from build123d import *

# Parameters (mm, degrees)
EXTRUDE_1_DEPTH           = 70
SKETCH_4_R                = 2.5
EXTRUDE_2_DEPTH           = 10
M5X0_8_TAPPED_HOLE1_D     = 4.2
M5X0_8_TAPPED_HOLE1_DEPTH = 12.4
M5X0_8_TAPPED_HOLE1_TIP   = 1.2618073


with BuildPart() as part:
    # 草圖1 → 填料-伸長1 (new body)
    with BuildSketch(Plane.XY):
        Polygon((-2.020725942, 3.5), (-4.041451884, 0), (-2.020725942, -3.5), (2.020725942, -3.5), (4.041451884, 0), (2.020725942, 3.5), align=None)
    extrude(amount=EXTRUDE_1_DEPTH)

    # 草圖4 → 填料-伸長2 (add)
    with BuildSketch(Plane(origin=(0, 0, 0), x_dir=(-1, 0, 0), z_dir=(0, 0, -1))):
        Circle(SKETCH_4_R)
    extrude(amount=EXTRUDE_2_DEPTH)

    # M5x0.8 Tapped Hole1
    with Locations(Plane.XY.offset(70)):
        with Locations((0, 0)):
            Hole(M5X0_8_TAPPED_HOLE1_D / 2, depth=M5X0_8_TAPPED_HOLE1_DEPTH)
            with Locations((0, 0, -(M5X0_8_TAPPED_HOLE1_DEPTH + M5X0_8_TAPPED_HOLE1_TIP / 2))):  # 118° drill point
                Cone(0, M5X0_8_TAPPED_HOLE1_D / 2, M5X0_8_TAPPED_HOLE1_TIP, mode=Mode.SUBTRACT)


solid = part.part
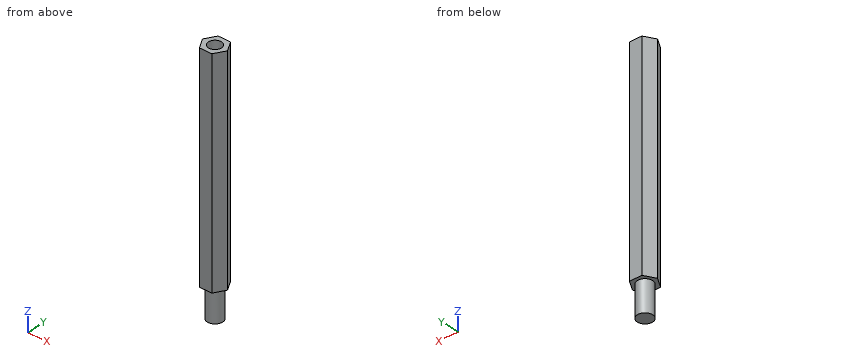
Part model, mm, in its own coordinate system. Coordinates: 2 decimals unless noted, no trailing zeros. Write each loop counter-clockwise with the first axis right and the second up, starting at its lowest first coordinate (ties: lowest second). Pieces come first, ordered by that corner, then holes. Notation, with made-up numbers: M 21,31 L 60,31 A12 cw 60,35 Z; hole C 65.25,49 d9. An arc over 180 degrees is marked long. Return JSON: item names as keys, results as strings.
1. Probe L1, parallel to Y at x = 0, z = 65.25; L2, parallel to X at y = 0, z = 61.75; L3, parallel to X at y = 1, z = 64.5. List the from-to ranges inside material, lowest first.
Determined:
{"L1": "-3.5 to -2.1, 2.1 to 3.5", "L2": "-4.04 to -2.1, 2.1 to 4.04", "L3": "-3.46 to -1.85, 1.85 to 3.46"}
2. Flat gauge pins, fed straight in: pin 1 Ø1.5 at (y, z) = (2.5, 16.5) entering from -X; pin 2 Ø3.5 at (x, y) = (0, 0) entering from +Z; pin 3 Ø3 at (y, z) = (-2.5, 11.5) entering from -X. Where does each tip first touch, or does it go through?
Determined:
{"pin 1": "x = -3.03", "pin 2": "z = 57.39", "pin 3": "x = -3.46"}
3. Saw through at A-A, the plane z = 12. Write the cut outline in (x, y).
Determined:
{"outline": "M -4.04,0 L -2.02,-3.5 L 2.02,-3.5 L 4.04,0 L 2.02,3.5 L -2.02,3.5 Z"}
